```python
from build123d import *
from build123d.topology import SkipClean

# Parameters (mm, degrees)
CROQUIS1_R                 = 17.1
CROQUIS1_R_2               = 14.1
SALIENTE_EXTRUIR1_DEPTH    = 7.5
CORTAR_EXTRUIR1_REACH      = 30.457
CROQUIS2_W                 = 15.420651877
CROQUIS2_H                 = 7.2
CROQUIS54_W                = 3
CROQUIS54_H                = 25
REVOLUCI_N1_ANGLE          = 150
CORTAR_BARRER2_PROFILE_R   = 2.25
CHAFL_N3_SIZE              = 5
CORTAR_EXTRUIR2_REACH      = 29.223
CORTAR_EXTRUIR2_END_RADIUS = 16.1
CROQUIS61_R                = 3
CORTAR_EXTRUIR3_START      = -17.1
CORTAR_EXTRUIR3_DEPTH      = 33.816758059
CROQUIS63_R                = 0.75
CORTAR_EXTRUIR4_DEPTH      = 10
CROQUIS64_R                = 1.25
CORTAR_EXTRUIR5_DEPTH      = 0.6
CORTAR_EXTRUIR6_START      = -6
CROQUIS65_W                = 2.8
CROQUIS65_H                = 19.872981168
CORTAR_EXTRUIR6_DEPTH      = 11


# Read off the part's stored shape, not the designer's step: Cortar-Extruir3
with BuildPart() as part:
    # Croquis1 → Saliente-Extruir1 (new, symmetric)
    with BuildSketch(Plane(origin=(0, 0, 0), x_dir=(1, 0, 0), z_dir=(0, 1, 0))):
        with Locations(Location((0, 0, 0), (0, 0, 270))):
            Circle(CROQUIS1_R)
        with Locations(Location((0, 0, 0), (0, 0, 270))):
            Circle(CROQUIS1_R_2, mode=Mode.SUBTRACT)
    extrude(amount=SALIENTE_EXTRUIR1_DEPTH, both=True)

    # Croquis2 → Cortar-Extruir1 (cut, up to next)
    with BuildSketch(Plane(origin=(0, 7.5, 0), x_dir=(1, 0, 0), z_dir=(0, 1, 0)), mode=Mode.PRIVATE) as cortar_extruir1_sk1:
        with Locations((15.870282115, 0)):
            Rectangle(CROQUIS2_W, CROQUIS2_H)
    cortar_extruir1_tool1 = extrude(cortar_extruir1_sk1.sketch, amount=-CORTAR_EXTRUIR1_REACH, mode=Mode.PRIVATE) & part.part
    add(cortar_extruir1_tool1.solids().sort_by_distance((15.870282, 7.5, 0))[0], mode=Mode.SUBTRACT)

    # Croquis54 → Revolución1 (revolve, symmetric)
    with SkipClean():  # the faces are left unmerged after this step: merging them gives an invalid solid
        with BuildSketch(Plane.XY) as revoluci_n1_sk:
            with Locations((-15.6, 0)):
                Rectangle(CROQUIS54_W, CROQUIS54_H)
        revolve(axis=Axis((0, -13.582020258, 0), (0, 1, 0)), revolution_arc=REVOLUCI_N1_ANGLE / 2)
        revolve(revoluci_n1_sk.sketch, axis=Axis((0, -13.582020258, 0), (0, -1, 0)), revolution_arc=REVOLUCI_N1_ANGLE / 2)
    add(part.part.scale(1), mode=Mode.REPLACE)  # the faces are merged on a copy

    # Cortar-Barrer2: sweep along a path in Croquis12
    with BuildLine(Plane(origin=(0, 0, 0), x_dir=(1, 0, 0), z_dir=(0, 1, 0))) as cortar_barrer2_path:
        CenterArc((0, 0), 14.1, 0, 360)
    # Cortar-Barrer2 profile (on start of the path) → Cortar-Barrer2 (sweep, cut)
    with BuildSketch(Plane(origin=(14.1, 0, 0), x_dir=(-1, 0, 0), z_dir=(0, 0, -1))):
        Circle(CORTAR_BARRER2_PROFILE_R)
    sweep(path=cortar_barrer2_path.line, mode=Mode.SUBTRACT)

    # Chaflán3
    chafl_n3_edges = [part.edges().sort_by_distance(p)[0] for p in [
        (-4.037577104, -12.5, -15.06844289),
        (-4.037577104, 12.5, -15.06844289),
        (-4.037577104, -12.5, 15.06844289),
        (-4.037577104, 12.5, 15.06844289),
    ]]
    chamfer(chafl_n3_edges, length=CHAFL_N3_SIZE - 0.0001)  # a hair under: the kernel refuses the full size

    # Cortar-Extruir2: up to this cylinder (the profile starts inside it)
    cortar_extruir2_end = Plane(origin=(0, 0, 0), z_dir=(0, -1, 0)) * Cylinder(CORTAR_EXTRUIR2_END_RADIUS, 91.646, mode=Mode.PRIVATE)
    # Croquis61 → Cortar-Extruir2 (cut, up to the surface)
    with BuildSketch(Plane(origin=(0, 0, 0), x_dir=(0, 0, -1), z_dir=(1, 0, 0)), mode=Mode.PRIVATE) as cortar_extruir2_sk1:
        Circle(CROQUIS61_R)
    cortar_extruir2_tool1 = extrude(cortar_extruir2_sk1.sketch, amount=-CORTAR_EXTRUIR2_REACH, mode=Mode.PRIVATE) & cortar_extruir2_end
    add(cortar_extruir2_tool1.solids().sort_by_distance((0, 0, 0))[0], mode=Mode.SUBTRACT)

    # Cortar-Extruir3 outline → Cortar-Extruir3 (cut)
    with BuildSketch(Plane(origin=(0, 0, 0), x_dir=(0, 0, -1), z_dir=(1, 0, 0)).offset(CORTAR_EXTRUIR3_START)):
        Polygon((3.6, 0), (-3.6, 0), (-3.6, 1.5), (-20.692074401, 1.5), (-20.692074401, -12.752391624), (19.353781031, -12.752391624), (19.353781031, 1.5), (3.6, 1.5), align=None)
    extrude(amount=CORTAR_EXTRUIR3_DEPTH, mode=Mode.SUBTRACT)

    # Croquis63 → Cortar-Extruir4 (cut)
    with SkipClean():  # the faces are left unmerged after this step: merging them gives an invalid solid
        with BuildSketch(Plane(origin=(-17.1, 0, 0), x_dir=(0, -1, 0), z_dir=(-1, 0, 0))):
            with Locations(Location((-5.5, 0, 0), (0, 0, 90))):
                Circle(CROQUIS63_R)
        extrude(amount=-CORTAR_EXTRUIR4_DEPTH, mode=Mode.SUBTRACT)

    # Croquis64 → Cortar-Extruir5 (cut)
    with SkipClean():  # the faces are left unmerged after this step: merging them gives an invalid solid
        with BuildSketch(Plane(origin=(-17.1, 0, 0), x_dir=(0, -1, 0), z_dir=(-1, 0, 0))):
            with Locations(Location((-5.5, 0, 0), (0, 0, 90))):
                Circle(CROQUIS64_R)
        extrude(amount=-CORTAR_EXTRUIR5_DEPTH, mode=Mode.SUBTRACT)

    # Croquis65 → Cortar-Extruir6 (cut)
    with SkipClean():  # the faces are left unmerged after this step: merging them gives an invalid solid
        with BuildSketch(Plane(origin=(0, 7.5, 0), x_dir=(1, 0, 0), z_dir=(0, 1, 0)).offset(CORTAR_EXTRUIR6_START)):
            with Locations((15.316758059, 0)):
                Rectangle(CROQUIS65_W, CROQUIS65_H)
        extrude(amount=CORTAR_EXTRUIR6_DEPTH, mode=Mode.SUBTRACT)


solid = part.part
```
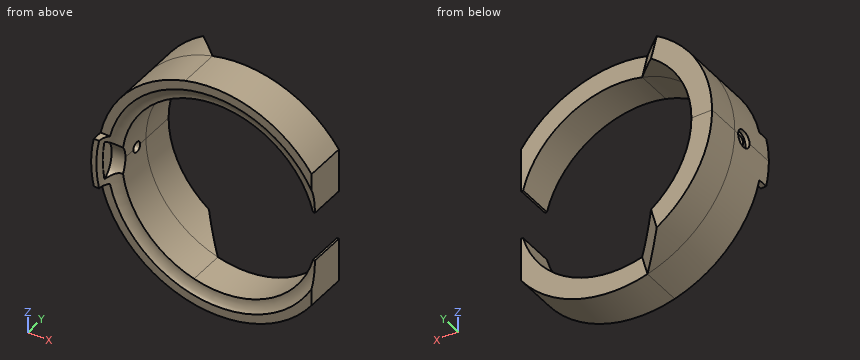
The model under review builds one solid part; all positions refer to its coordinate system, in mm. Round coordinates to 2 decimals unless told otherwise and drop trailing zeros. Loops run counter-clockwise (first coordinate to the right, second up) from the corner with the lowest first, then second, coordinate; pieces in that order, holes last. Notation, with made-up numbers: M 11.5,74 L 47.5,74 A22 cw 47.5,88 Z; hole C -24.75,57 d3. An arc over 180 degrees is marked long. Answer as a JSON object with one key per item and string values.
(1) To check wall thickness, follow line 1 along Y through (x, z) = (-16.8, 0); line 2 along Y through (x, z) = (-15.8, 0); line 3 along X through (y, z) = (2.25, -0.5). State the ranges of each line that lie inside material, in increasing order.
Resolved:
{"line 1": "0 to 4.25, 6.75 to 12.5", "line 2": "3 to 4.75, 6.25 to 12.5", "line 3": "-17.09 to -16.09"}
(2) Take a section at C-C on y = 11. Give the boundary of the cut face in (x, z).
Resolved:
{"outline": "M -7.71,-15.26 L -6.92,-12.29 A14.1 cw -6.92,12.29 L -7.71,15.26 A17.1 ccw Z"}
(3) Take a section at A-A on y = 5.5. Give the boundary of the cut face in (x, z).
Resolved:
{"outline": "M -17.05,-1.25 A17.1 ccw 13.92,-9.94 L 13.92,-3.6 L 13.63,-3.6 A14.1 cw -14.08,-0.75 L -16.5,-0.75 L -16.5,-1.25 Z; M -17.05,1.25 L -16.5,1.25 L -16.5,0.75 L -14.08,0.75 A14.1 cw 13.63,3.6 L 13.92,3.6 L 13.92,9.94 A17.1 ccw Z"}
(4) Clearance check with flat-ended pins moving along their axes: P1, Ø1.2, axis at y = 5.5, z = 0, coming from the -X side; P2, Ø11, axis at x = -8, z = 12, coming from the -Y side; P3, Ø5, axis at x = 11, y = 4.5, coming from the +Z side; P4, Ø1.5, axis at x = -14, z = 4, coming from the -Y side. State where each tip first meets the part, or that it passes through.
Resolved:
{"P1": "through", "P2": "y = 1.5", "P3": "z = 14.84", "P4": "y = 1.9"}
(5) Take a section at B-B on y = 3.5. Give the boundary of the cut face in (x, z).
Resolved:
{"outline": "M 13.63,-3.6 A14.1 cw long 13.63,3.6 L 13.92,3.6 L 13.92,9.94 A17.1 ccw long 13.92,-9.94 L 13.92,-3.6 Z"}
(6) Take a section at D-D on y = 8. Give the boundary of the cut face in (x, z).
Resolved:
{"outline": "M -4.91,-16.38 L -4.13,-13.48 A14.1 cw -4.13,13.48 L -4.91,16.38 A17.1 ccw Z"}
